Source: CAD feature listing. Evaluate the final solid. Frame: model axes, mm. A direction names the side the tool comes from. Round coordinates to 2 decimals unless told otherwise and drop trailing zeros. Write each loop counter-clockwise with the first axis right and the second up, starting at its lowest first coordinate (ties: lowest second). Pieces come first, ordered by that corner, then holes. Notation, with made-up numbers: M 80,70 L 110,70 A11 cw 110,85 Z; hole C 55.25,23 d5. An arc over 180 degrees is marked long. Answer in a Markdown table with one row per item. Add a question column.
Item 1: Material intervals for probe 1 along Y at (x, z) = (14.5, 0.3); probe 2 along Y at (x, z) = (33.5, 1.35); probe 3 along X at (y, z) = (6.5, 3.1), sorted ascending.
Item 2: Cut plane D-D on y = 11. Return loops of the section in (x, z).
Item 3: Cut plane A-A on z = 3.05. Return loops of the section in (x, y), and give its area (3 significant figures).
Item 4: Cut plane C-C on x = 10.5. Return loops of the section in (y, z).
Item 5: Cut plane B-B on x = 28. Return loops of the section in (y, z).
Item 6: Mould query, pull axis X, two halves, no side actions, for faces 1 (the face through (39.327, -34.714, 2.46)), 2 (the face through (-2, -2, 4.99)), 3 (the face through (-28.597, -2, 2)). Classes: released by +X, released by -X, zero draft, split by the parting line, or undercut.
Item 7: Set-up query: faces 4 (the face through (36.403, 43, 2)), 5 (the face through (34.59, 33.51, 2.46)), 6 (the face through (4, 47.02, 2)). Return all of +Z, -Z, +X, -X, +Y, -Y with unobstructed straight access to the full face (end or side cutting, diameter ignored); none if empty.
Item 8: Contact query for flat-ended pins moving along their axis: pin 1 (1 mm diameter, centred on x = 15.5, y = -25.5, fed in from -Z); pin 2 (2 mm diameter, centred on y = -5, z = 1.5, fed in from +X). Output: stop coordinate, or through.
from build123d import *

# Parameters (mm, degrees)
F1_DEPTH = 4.99


with BuildPart() as f1:
    # F0 (on Top) → F1 (new body)
    with BuildSketch(Plane.XY):
        with BuildLine():
            Line((36.402646, 47.020067), (-28.597354, 47.020067))
            Line((-28.597354, 47.020067), (-28.597354, -52.979933))
            Line((-28.597354, -52.979933), (41.402646, -52.979933))
            Line((41.402646, -52.979933), (41.402646, -40.812817))
            ThreePointArc((41.402646, -40.812817), (39.270242, -34.640222), (33.782461, -31.10012))
            ThreePointArc((33.782461, -31.10012), (9.444835, -1.995757), (29.972369, 29.910424))
            ThreePointArc((29.972369, 29.910424), (34.639673, 33.581354), (36.402646, 39.251574))
            Line((36.402646, 39.251574), (36.402646, 47.020067))
        make_face()
    extrude(amount=F1_DEPTH)


solid = f1.part
Results below:
| question | item | result |
|---|---|---|
| 1 | probe 1 | -52.98 to -17.36, 17.36 to 47.02 |
| 1 | probe 2 | -52.98 to -31.03, 32.21 to 47.02 |
| 1 | probe 3 | -28.6 to 10.05 |
| 2 | outline | M -28.6,0 L 11.33,0 L 11.33,4.99 L -28.6,4.99 Z |
| 3 | outline | M -28.6,-52.98 L 41.4,-52.98 L 41.4,-40.81 A10 ccw 33.78,-31.1 A32.02 cw 29.97,29.91 A10 ccw 36.4,39.25 L 36.4,47.02 L -28.6,47.02 Z |
| 3 | area | 5,290 mm2 |
| 4 | outline | M -52.98,0 L -8.39,0 L -8.39,4.99 L -52.98,4.99 Z; M 8.39,0 L 47.02,0 L 47.02,4.99 L 8.39,4.99 Z |
| 5 | outline | M -52.98,0 L -29.08,0 L -29.08,4.99 L -52.98,4.99 Z; M 29.08,0 L 47.02,0 L 47.02,4.99 L 29.08,4.99 Z |
| 6 | face 1 | released by +X |
| 6 | face 2 | zero draft |
| 6 | face 3 | released by -X |
| 7 | face 4 | +Z, -Z, +X, +Y |
| 7 | face 5 | +Z, -Z, +X |
| 7 | face 6 | +Z, -Z, +X, -X, +Y |
| 8 | pin 1 | z = 0 |
| 8 | pin 2 | x = 9.95 |
